The model under review builds one solid part; all positions refer to its coordinate system, in mm. A direction names the side the tool comes from. Coordinates: 2 decimals unless noted, no trailing zeros. Loops run counter-clockwise (first coordinate to the right, second up) from the corner with the lowest first, then second, coordinate; pieces in that order, holes last. Notation, with made-up numbers: (53.5, 86.25) - (103.5, 86.25) arc R10 cw to (103.5, 99.25) - close; hole circle Ø2 at (-19.5, -18). An arc over 180 degrees is marked (long way). Answer in a Markdown table with one row per item. Add a question column.
(1) We need section B-B on y = -7. Write out the cut boundary in (x, z), plus the area to 3 significant figures.
(2) We need section C-C on x = -6. Write out the cut boundary in (y, z).
(3) Machinability: for faces 1 (the flat face through (-26.136, -2, 5)), 2 (the flat face through (-10.05, -5.13, 4.93)), which of the approach directions +Z, -Z, +X, -X, +Y, -Y give a long, thin tool a straight path to every point of the face, cutting with its end or side? Answer none if there is none.
(4) For line 1 along X through (y, z) = (6, 8.75); line 2 along X through (y, z) = (0.25, 7); line 3 along Y through (x, z) = (-9, 7.5), list the stretches that pass through material, from the lowest coordinate up.
(5) For P1, Ø12, axis at x = -13.5, y = 4, coming from the -Z side, flat-tipped, find the tip position at first contact; note if it passes through.
(6) We need section A-A on z = 3.25. Write out the cut boundary in (x, y).
(7) Mouldability with a two-part tool opening along Y and no side actions: class faces 3 (the flat face through (-11, -14.206, 5)), 4 (the flat face through (-11, 10.794, 5)), 5 (the flat face through (-10.31, 2.37, 4.93)) as +Y half, -Y half, draft (parallel to the pull), parting line (faces both ways), or undercut.
from build123d import *

# Parameters (mm, degrees)
F0_W     = 30
F0_H     = 25
F1_DEPTH = 10


with BuildPart() as f1:
    # F0 (on Top) → F1 (new body)
    with BuildSketch(Plane.XY):
        with Locations((-11.136306, -1.705752)):
            Rectangle(F0_W, F0_H)
        Polygon((-19.450465, -8.932962), (-19.450465, 6.067038), (-0.909969, -1.432962), align=None, mode=Mode.SUBTRACT)
    extrude(amount=F1_DEPTH)


solid = f1.part
Outcome:
| question | item | result |
|---|---|---|
| 1 | outline | (-26.14, 0) - (-19.45, 0) - (-19.45, 10) - (-26.14, 10) - close; (-14.67, 0) - (3.86, 0) - (3.86, 10) - (-14.67, 10) - close |
| 1 | area | 252 mm² |
| 2 | outline | (-14.21, 0) - (-3.49, 0) - (-3.49, 10) - (-14.21, 10) - close; (0.63, 0) - (10.79, 0) - (10.79, 10) - (0.63, 10) - close |
| 3 | face 1 | +Z, -Z, -X, +Y, -Y |
| 3 | face 2 | +Z, -Z |
| 4 | line 1 | -26.14 to -19.45, -19.28 to 3.86 |
| 4 | line 2 | -26.14 to -19.45, -5.07 to 3.86 |
| 4 | line 3 | -14.21 to -4.71, 1.84 to 10.79 |
| 5 | P1 | z = 0 |
| 6 | outline | (-26.14, -14.21) - (3.86, -14.21) - (3.86, 10.79) - (-26.14, 10.79) - close; hole (-19.45, -8.93) - (-0.91, -1.43) - (-19.45, 6.07) - close |
| 7 | face 3 | -Y half |
| 7 | face 4 | +Y half |
| 7 | face 5 | undercut |
